```python
from build123d import *

# Parameters (mm, degrees)
F0_W        = 100
F0_H        = 50
F1_DEPTH    = 25
F2_T        = -4
F3_T1_DEPTH = 75
F3_T3_DEPTH = 125


# Not quite as in the source:
# - a fillet or chamfer that OpenCascade refuses, or shapes differently, is made with other operations: its cross-section is extruded or revolved along the edge and cut away or added


with BuildPart() as f1:
    # F0 (on Top) → F1 (new body)
    with BuildSketch(Plane.XY):
        with Locations((-4.7528631985, -11.9245312498)):
            Rectangle(F0_W, F0_H)
    extrude(amount=F1_DEPTH)

    # F2
    f2_openings = [f1.faces().sort_by_distance(p)[0] for p in [
        (-4.752863, -11.924531, 25),
    ]]
    offset(amount=F2_T, openings=f2_openings)

    # F3: fillet of radius 5 on 4 edges, made by hand

    # F3_s2 → F3_t1 (cut)
    with BuildSketch(Plane.XZ.offset(-25.5754687502)):
        with BuildLine():
            ThreePointArc((-54.7528631985, 20), (-53.2883971045, 23.5355339059), (-49.7528631985, 25))
            Line((-49.7528631985, 25), (-54.7528631985, 25))
            Line((-54.7528631985, 25), (-54.7528631985, 20))
        make_face()
        with BuildLine():
            ThreePointArc((45.2471368015, 20), (43.7826707074, 23.5355339059), (40.2471368015, 25))
            Line((40.2471368015, 25), (45.2471368015, 25))
            Line((45.2471368015, 25), (45.2471368015, 20))
        make_face()
    extrude(amount=F3_T1_DEPTH, mode=Mode.SUBTRACT)

    # F3_s4 → F3_t3 (cut)
    with BuildSketch(Plane.YZ.offset(-67.2528631985)):
        with BuildLine():
            ThreePointArc((13.0754687502, 20), (11.6110026561, 23.5355339059), (8.0754687502, 25))
            Line((8.0754687502, 25), (13.0754687502, 25))
            Line((13.0754687502, 25), (13.0754687502, 20))
        make_face()
        with BuildLine():
            ThreePointArc((-36.9245312498, 20), (-35.4600651557, 23.5355339059), (-31.9245312498, 25))
            Line((-31.9245312498, 25), (-36.9245312498, 25))
            Line((-36.9245312498, 25), (-36.9245312498, 20))
        make_face()
    extrude(amount=F3_T3_DEPTH, mode=Mode.SUBTRACT)


solid = f1.part
```
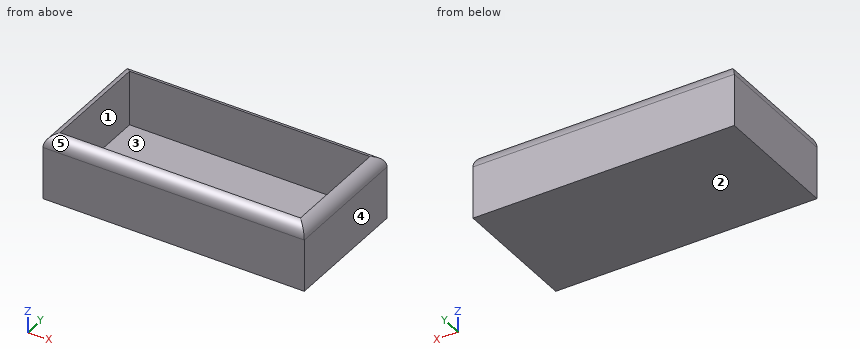
Geometry: final body of the model. Coordinates: model frame, mm. Face numbers are marked on the shaded views. A direction names the side the tool comes from. Coordinates: 2 decimals unless noted, no trailing zeros. Order: outer loops, then holes, each group sorted by start corner. A loop starts at its lowest first (then second) coordinate and runs counter-clockwise, first axis right, second up. Notation, with made-up numbers: (-13, -5) - (23, -5) arc R6 cw to (23, 0) - close; hole circle Ø5 at (30.25, 83). An arc over 180 degrees is marked (long way). Write each question's results on one line, items separated by ' | '.
1) Set-up query: the marked faces 1 and 2. Return all of +Z, -Z, +X, -X, +Y, -Y with unobstructed straight access to the full face (end or side cutting, diameter ignored); none if empty.
Results list:
face 1: +Z | face 2: -Z, +X, -X, +Y, -Y
2) Line query: line 1 (X direction, y = -20.5, z = 16.5); line 2 (Y direction, x = -2.5, z = 8); line 3 (Y direction, x = -27.5, z = 21.5). Output: solid intervals per line, ascending. Write a range as from..to.
Results list:
line 1: -54.75..-50.75, 41.25..45.25 | line 2: -36.92..-32.92, 9.08..13.08 | line 3: -36.69..-32.92, 9.08..12.85
3) Section B-B, the plane y = 1.5. Return loops of the section in (x, z), plus the area to 3 significant figures.
Results list:
outline: (-54.75, 0) - (45.25, 0) - (45.25, 20) arc R5 ccw to (41.25, 24.9) - (41.25, 4) - (-50.75, 4) - (-50.75, 24.9) arc R5 ccw to (-54.75, 20) - close | area: 557 mm^2
4) Section C-C, the plane x = -7.5. Return loops of the section in (y, z).
Results list:
outline: (-36.92, 0) - (13.08, 0) - (13.08, 20) arc R5 ccw to (9.08, 24.9) - (9.08, 4) - (-32.92, 4) - (-32.92, 24.9) arc R5 ccw to (-36.92, 20) - close
5) Section D-D, the plane z = 21.25. Return loops of the section in (x, y), plus the area to 3 significant figures.
Results list:
outline: (-54.59, -36.77) - (45.09, -36.77) - (45.09, 12.92) - (-54.59, 12.92) - close; hole (-50.75, -32.92) - (41.25, -32.92) - (41.25, 9.08) - (-50.75, 9.08) - close | area: 1,090 mm^2
6) Section A-A, the plane z = 11.75. Return loops of the section in (x, y), plus the area to 3 significant figures.
Results list:
outline: (-54.75, -36.92) - (45.25, -36.92) - (45.25, 13.08) - (-54.75, 13.08) - close; hole (-50.75, -32.92) - (41.25, -32.92) - (41.25, 9.08) - (-50.75, 9.08) - close | area: 1,140 mm^2
7) Pin query (flat end, axial travel): pin 1 (1 mm diameter, centred on y = -12.5, z = 21, fed in from -X); pin 2 (21 mm diameter, centred on x = 8, y = -19, fed in from +Z). Return the tip coordinate at first contact, or that it passes through.
Results list:
pin 1: x = -54.73 | pin 2: z = 4
8) Pull-direction query (X, two-part tool) for the marked faces 3, 4 and 5; classes: pulls with the +X half, pulls with the -X half, needs draft (parallel to the pull), parting line crosses it, or undercut.
Results list:
face 3: undercut | face 4: pulls with the +X half | face 5: needs draft
